Drawing for the job (mm, zero at the part's lowest x, y, z). A direction names the side the tool comes from. Coordinates: 2 decimals unless noted, no trailing zeros. Write each loop counter-clockwise with the first axis right and the second up, starting at its lowest first coordinate (ties: lowest second). Pieces come first, ordered by that corner, then holes. Notation, with made-up numbers: M 55.25,49 L 85.25,49 A25 cw 85.25,79 Z; hole C -19,77.25 d7. An arc over 180 degrees is marked long. Put each result on its own line as item: value. Start each with the question number.
Q1. Cut at A-A (z = 62). Write the cut outline in (x, y), then the cut area to 3 significant figures.
Q2. Which spindle directions (+Z, -Z, +X, -X, +Y, -Y) get a long thin tool onto all of the face, cutting with end or side? Do the marked faces 4 and 5. Say none if no direction does.
Q3. Pull direction X, two halves, no side cores. Call the marked faces 1, 2 and 3: pulls with the +X half, pulls with the -X half, needs draft (parallel to the pull), parting line crosses it, or undercut.
Q4. Drill centre lines: line 1 along Z through (x, y) = (79.5, 163) (1 decimal); line 2 along X through (y, z) = (49, 113). Where is each one in solid material? Low to high.
Q5. Cut at B-B (x = 75.5). Write the cut outline in (y, z) (1 decimal), then the cut area to 3 significant figures.
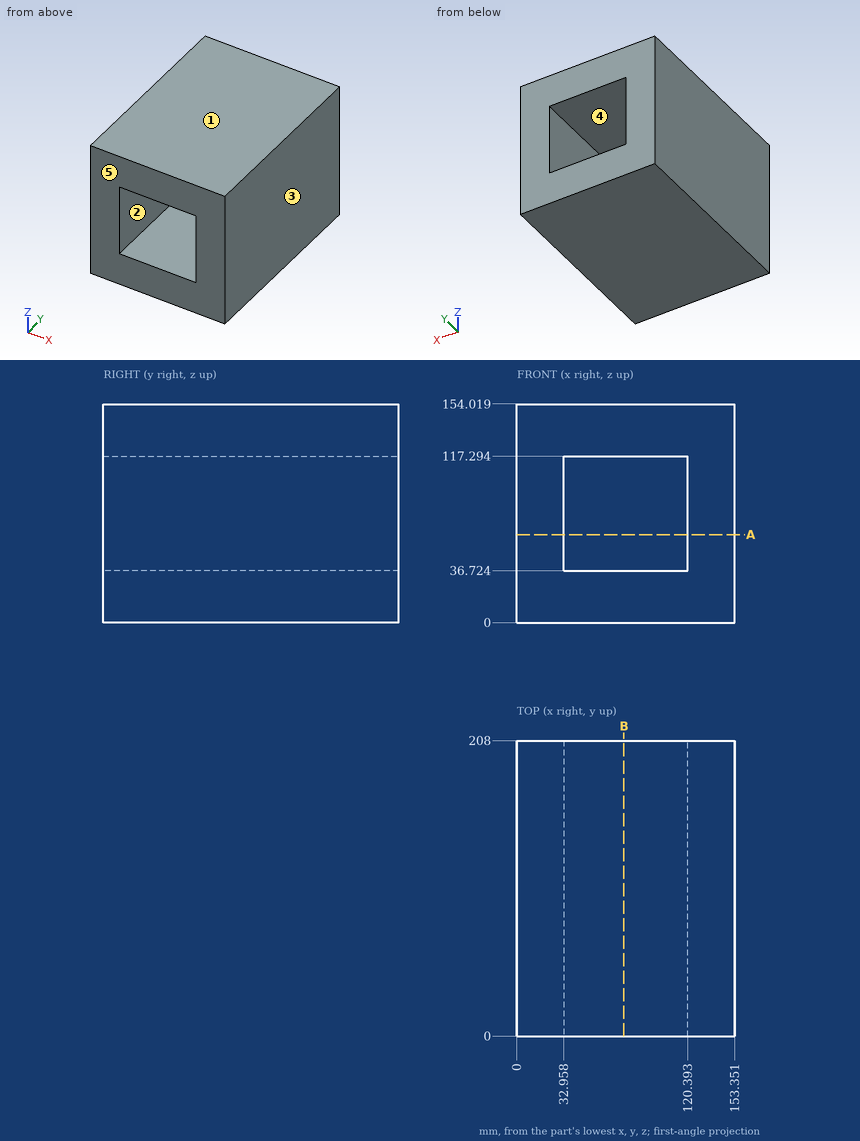
Computed values:
1. outline: M 0,0 L 32.96,0 L 32.96,208 L 0,208 Z; M 120.39,0 L 153.35,0 L 153.35,208 L 120.39,208 Z
1. area: 13,700 mm2
2. face 4: +Y, -Y
2. face 5: +Z, -Z, +X, -X, -Y
3. face 1: needs draft
3. face 2: undercut
3. face 3: pulls with the +X half
4. line 1: 0 to 36.7, 117.3 to 154
4. line 2: 0 to 32.96, 120.39 to 153.35
5. outline: M 0,0 L 208,0 L 208,36.7 L 0,36.7 Z; M 0,117.3 L 208,117.3 L 208,154 L 0,154 Z
5. area: 15,300 mm2
